```python
from build123d import *

# Parameters (mm, degrees)
BOSS_EXTRUDE1_DEPTH      = 8.7806917
BOSS_EXTRUDE1_DEPTH_BACK = 3
SKETCH1_R                = 8.175
SKETCH1_R_2              = 3.25
SKETCH1_3_R              = 14.023642089
SKETCH1_3_R_2            = 8.175
BOSS_EXTRUDE2_DEPTH      = 3
SKETCH2_R                = 2.5
CUT_EXTRUDE1_DEPTH       = 15
CUT_EXTRUDE2_DEPTH       = 3.175
CUT_EXTRUDE2_DEPTH_BACK  = 24.067504724
SKETCH3_R                = 1
SKETCH4_R                = 4.175
BOSS_EXTRUDE4_DEPTH      = 5
CUT_EXTRUDE3_DEPTH       = 15
CUT_EXTRUDE3_DEPTH_BACK  = 13
SKETCH1_5_R              = 3.25


with BuildPart() as part:
    # Sketch1 → Boss-Extrude1 (new, two sides: drawn at the far end of the back side and taken through both)
    with BuildSketch(Plane(origin=(0, 0, 0), x_dir=(1, 0, 0), z_dir=(0, 1, 0)).offset(-BOSS_EXTRUDE1_DEPTH_BACK)):
        with Locations(Location((0, 0, 0), (0, 0, 270))):
            Circle(SKETCH1_R)
        with Locations(Location((0, 0, 0), (0, 0, 270))):
            Circle(SKETCH1_R_2, mode=Mode.SUBTRACT)
    extrude(amount=BOSS_EXTRUDE1_DEPTH + BOSS_EXTRUDE1_DEPTH_BACK)

    # Sketch2 → Cut-Extrude1 (cut)
    with BuildSketch(Plane(origin=(0, 0, 0), x_dir=(0, 0, -1), z_dir=(1, 0, 0))):
        with Locations((0, 4.5)):
            Circle(SKETCH2_R)
    extrude(amount=-CUT_EXTRUDE1_DEPTH, mode=Mode.SUBTRACT)



with BuildPart() as body_2:
    # Sketch1_3 → Boss-Extrude2 (new body)
    with BuildSketch(Plane(origin=(0, 0, 0), x_dir=(1, 0, 0), z_dir=(0, 1, 0))):
        with Locations(Location((0, 0, 0), (0, 0, 270))):
            Circle(SKETCH1_3_R)
        with Locations(Location((0, 0, 0), (0, 0, 270))):
            Circle(SKETCH1_3_R_2, mode=Mode.SUBTRACT)
    extrude(amount=-BOSS_EXTRUDE2_DEPTH)

    # Sketch3 → Cut-Extrude2 (cut, two sides: drawn at the far end of the back side and taken through both)
    with BuildSketch(Plane.XZ.offset(3).offset(-CUT_EXTRUDE2_DEPTH_BACK)):
        with Locations(Location((0, 11.797323524, 0), (0, 0, 90))):
            Circle(SKETCH3_R)
        with Locations(Location((9.22351894, 7.355510906, 0), (0, 0, 90))):
            Circle(SKETCH3_R)
        with Locations(Location((11.501539993, -2.625151449, 0), (0, 0, 90))):
            Circle(SKETCH3_R)
        with Locations(Location((5.118666842, -10.62902122, 0), (0, 0, 90))):
            Circle(SKETCH3_R)
        with Locations(Location((-5.118666842, -10.62902122, 0), (0, 0, 90))):
            Circle(SKETCH3_R)
        with Locations(Location((-11.501539993, -2.625151449, 0), (0, 0, 90))):
            Circle(SKETCH3_R)
        with Locations(Location((-9.22351894, 7.355510906, 0), (0, 0, 90))):
            Circle(SKETCH3_R)
    extrude(amount=CUT_EXTRUDE2_DEPTH + CUT_EXTRUDE2_DEPTH_BACK, mode=Mode.SUBTRACT)


with BuildPart() as part_1:
    add(part.part)

    add(body_2.part)  # Boss-Extrude4 merges body 2
    # Sketch4 → Boss-Extrude4 (add)
    with BuildSketch(Plane.XZ.offset(3)):
        with Locations(Location((0, 0, 0), (0, 0, 90))):
            Circle(SKETCH4_R)
    extrude(amount=BOSS_EXTRUDE4_DEPTH)

    # Sketch1_5 → Cut-Extrude3 (cut, two sides: drawn at the far end of the back side and taken through both)
    with BuildSketch(Plane(origin=(0, 0, 0), x_dir=(1, 0, 0), z_dir=(0, 1, 0)).offset(-CUT_EXTRUDE3_DEPTH_BACK)):
        with Locations(Location((0, 0, 0), (0, 0, 270))):
            Circle(SKETCH1_5_R)
    extrude(amount=CUT_EXTRUDE3_DEPTH + CUT_EXTRUDE3_DEPTH_BACK, mode=Mode.SUBTRACT)


solid = part_1.part
```
Geometry check sheet. Reference: the model listing, model coordinates, mm. A direction names the side the tool comes from. Give positions to 0.01 mm unless a question says otherwise; leave off trailing zeros. Write each loop counter-clockwise with the first axis right and the second up, starting at its lowest first coordinate (ties: lowest second). Pieces come first, ordered by that corner, then holes. Notation, with made-up numbers: (84, 79) -> (105, 79) arc R19 ccw to (105, 116) -> close; hole circle Ø7 at (36, -1). An arc over 180 degrees is marked (long way). Use one line per item in the form item = value.
Item 1: Sectioned sample at A-A on z = 0. Enter the section's corners in (x, y) (3 decimals).
Results list:
outline = (-14.024, -3) -> (-4.175, -3) -> (-4.175, -8) -> (-3.25, -8) -> (-3.25, 2) -> (-8.175, 2) -> (-8.175, 0) -> (-14.024, 0) -> close; (-8.175, 7) -> (-3.25, 7) -> (-3.25, 8.781) -> (-8.175, 8.781) -> close; (3.25, -8) -> (4.175, -8) -> (4.175, -3) -> (14.024, -3) -> (14.024, 0) -> (8.175, 0) -> (8.175, 8.781) -> (3.25, 8.781) -> close
Item 2: Sectioned sample at B-B on x = 0. Enter the section's corners in (y, z) (3 decimals).
Results list:
outline = (-8, -4.175) -> (-3, -4.175) -> (-3, -14.024) -> (0, -14.024) -> (0, -8.175) -> (8.781, -8.175) -> (8.781, -3.25) -> (-8, -3.25) -> close; (-8, 3.25) -> (8.781, 3.25) -> (8.781, 8.175) -> (0, 8.175) -> (0, 10.797) -> (-3, 10.797) -> (-3, 4.175) -> (-8, 4.175) -> close; (-3, 12.797) -> (0, 12.797) -> (0, 14.024) -> (-3, 14.024) -> close
Item 3: Sectioned sample at D-D on x = 7. Enter the section's corners in (y, z), plus the area to 3 significant figures.
Results list:
outline = (-3, -12.15) -> (0, -12.15) -> (0, -4.22) -> (8.78, -4.22) -> (8.78, 4.22) -> (0, 4.22) -> (0, 12.15) -> (-3, 12.15) -> close
area = 147 mm2
Item 4: Depth check by flat-ended pin: pin 1 Ø1.6 at (x, z) = (-9.22, 7.36) entering from -Y; pin 2 Ø10 at (x, z) = (-2.5, -9) entering from -Y; pin 3 Ø6 at (x, y) = (-7.5, -2.5) entering from +Z; pin 4 Ø6 at (x, z) = (-6.5, 7) entering from +Y. Enter the tip coordinate at first touch or a pass-through.
Results list:
pin_1 = through
pin_2 = -3
pin_3 = 13.28
pin_4 = 8.78
Item 5: Scan lines: line 1 (X direction, y = -0.75, z = 8); line 2 (X direction, y = -1.25, z = -2.5); line 3 (Y direction, x = -10.5, z = 9.25). Record each from-to range of solid material in increasing order.
Results list:
line_1 = -11.52 to -9.99, -8.46 to 8.46, 9.99 to 11.52
line_2 = -13.8 to -12.49, -10.51 to -2.08, 2.08 to 10.51, 12.49 to 13.8
line_3 = -3 to 0
Item 6: Sectioned sample at C-C on y = -2. Count the separate pieces of the cut face and the enclosed holes in it, plus the area to 3 significant figures.
Results list:
separate_pieces = 1
enclosed_holes = 8
area = 563 mm2
Item 7: Access from +Z, -Z, +X, -X, +Y, -Y to the whole of each face (thin tool, end or side, straight path). Record for faces 5 (the cylindrical face through (-10.525, -1.479, -2.842)), 6 (the cylindrical face through (-5.088, 5.251, -2.385)), 7 (the flat face through (-6, 0, 6)), 8 (the cylindrical face through (-1.254, -5.465, 3.982)).
Results list:
face_5 = +Y, -Y
face_6 = -X
face_7 = +Y
face_8 = -Y
Item 8: Mould release check, pull along X, two halves, no side actions. Record for faces 1 (the cylindrical face through (-4.51, -1.48, -11.42)), 2 (the flat face through (-2.9, -3, -3.3)), 3 (the cylindrical face through (6.893, 4.329, 4.395)), 4 (the cylindrical face through (12.48, -1.48, -2.84)): released by +X, released by -X, zero draft, split by the parting line, or undercut.
Results list:
face_1 = undercut
face_2 = zero draft
face_3 = split by the parting line
face_4 = undercut
